For this review, take the finished solid that the model builds, in its own axes (mm). A direction names the side the tool comes from. Give positions to 0.01 mm unless a question says otherwise; leave off trailing zeros. Write each loop counter-clockwise with the first axis right and the second up, starting at its lowest first coordinate (ties: lowest second). Pieces come first, ordered by that corner, then holes.
1) For P1, Ø3, axis at x = 5.5, z = 25, coming from the +Y side; P2, Ø12, axis at x = 18.5, y = 31.5, coming from the +Z side; P3, Ø11, axis at x = -6, z = 17, coming from the +Y side, all flat-tipped, find the tip position at first contact; note any pin that passes through.
2) Machinability: for faces 1 (the face through (34.38, 18.25, 19.14)), 2 (the face through (16, -76.2, 21)), 3 (the face through (38.1, -35, 11)), which of the approach directions +Z, -Z, +X, -X, +Y, -Y give a long, thin tool a straight path to every point of the face, cutting with its end or side? Answer none if there is none.
3) Wall thickness on line 1 along X through (y, z) = (43, 11.5); line 2 along Z through (x, y) = (4, -18); line 3 along Y through (x, z) = (-13, 43): over which ranges is each line inside the solid? List them lowest first.
4) We need section A-A on z = 33. Give the boundary of the cut face in (x, y).
5) We need section D-D on z = 17.5. Give the boundary of the cut face in (x, y), and give its area (3 significant figures).
from build123d import *

# Parameters (mm, degrees)
F0_W        = 88.9
F0_H        = 165.1
F1_DEPTH    = 6.35
F2_DEPTH    = 25.4
F3_DEPTH    = 50.8
F4_R        = 6.34999
F5_C1_SIZE2 = 12.7
F5_C1_SIZE  = 7.3323484187
F5_C2_SIZE2 = 7.3323484187
F5_C2_SIZE  = 12.7
F5_C3_SIZE2 = 7.3323484187
F5_C3_SIZE  = 12.7
F5_C4_SIZE2 = 7.3323484187
F5_C4_SIZE  = 12.7
F5_C5_SIZE2 = 7.3323484187
F5_C5_SIZE  = 12.7
F5_C6_SIZE2 = 7.3323484187
F5_C6_SIZE  = 12.7
F5_C7_SIZE2 = 12.7
F5_C7_SIZE  = 7.3323484187
F6_SIZE2    = 7.3323484187
F6_SIZE     = 12.7


# Not quite as in the source:
# - a fillet or chamfer is up to 0.001 mm smaller than in the source, because OpenCascade refuses the exact size


with BuildPart() as f1:
    # F0 (on Top) → F1 (new body)
    with BuildSketch(Plane.XY):
        Rectangle(F0_W, F0_H)
        Polygon((-38.1, 38.1), (-38.1, 76.2), (0, 76.2), (38.1, 76.2), (38.1, -38.1), (38.1, -76.2), (0, -76.2), (-38.1, -76.2), align=None, mode=Mode.SUBTRACT)
    extrude(amount=F1_DEPTH)

    # F0 (on Top) → F2 (join)
    with BuildSketch(Plane.XY):
        with BuildLine():
            Line((38.1, 76.2), (0, 76.2))
            Line((0, 76.2), (0, 50.8))
            ThreePointArc((0, 50.8), (-3.7197438789, 41.8197438789), (-12.7, 38.1))
            Line((-12.7, 38.1), (-38.1, 38.1))
            Line((-38.1, 38.1), (-38.1, -76.2))
            Line((-38.1, -76.2), (0, -76.2))
            Line((0, -76.2), (0, -50.8))
            ThreePointArc((0, -50.8), (3.7197438789, -41.8197438789), (12.7, -38.1))
            Line((12.7, -38.1), (38.1, -38.1))
            Line((38.1, -38.1), (38.1, 76.2))
        make_face()
    extrude(amount=F2_DEPTH)

    # F0 (on Top) → F3 (join)
    with BuildSketch(Plane.XY):
        with BuildLine():
            Line((38.1, -76.2), (38.1, -38.1))
            Line((38.1, -38.1), (12.7, -38.1))
            ThreePointArc((12.7, -38.1), (3.7197438789, -41.8197438789), (0, -50.8))
            Line((0, -50.8), (0, -76.2))
            Line((0, -76.2), (38.1, -76.2))
        make_face()
        with BuildLine():
            Line((0, 76.2), (-38.1, 76.2))
            Line((-38.1, 76.2), (-38.1, 38.1))
            Line((-38.1, 38.1), (-12.7, 38.1))
            ThreePointArc((-12.7, 38.1), (-3.7197438789, 41.8197438789), (0, 50.8))
            Line((0, 50.8), (0, 76.2))
        make_face()
    extrude(amount=F3_DEPTH)

    # F4 (radius 6.35 in the source; OpenCascade refuses exactly that, so slightly less here)
    f4_edges = [f1.edges().sort_by_distance(p)[0] for p in [
        (0, -82.55, 6.35),
        (44.45, 0, 6.35),
        (0, 82.55, 6.35),
        (-44.45, 0, 6.35),
    ]]
    fillet(f4_edges, radius=F4_R)

    # F5: chamfer of 12.7 x 7.3323484187 on 7 edges, made by hand

    # F5_c1
    f5_c1_edges = [f1.edges().sort_by_distance(p)[0] for p in [
        (-38.1, 57.15, 50.8),
    ]]
    f5_c1_side = f1.faces().sort_by_distance((-38.1, 57.15, 50.6533530316))[0]
    chamfer(f5_c1_edges, length=F5_C1_SIZE, length2=F5_C1_SIZE2, reference=f5_c1_side)

    # F5_c2
    f5_c2_edges = [f1.edges().sort_by_distance(p)[0] for p in [
        (-38.1, -19.05, 25.4),
    ]]
    f5_c2_side = f1.faces().sort_by_distance((-38.1, -19.05, 25.2533530316))[0]
    chamfer(f5_c2_edges, length=F5_C2_SIZE, length2=F5_C2_SIZE2, reference=f5_c2_side)

    # F5_c3
    f5_c3_edges = [f1.edges().sort_by_distance(p)[0] for p in [
        (19.05, 76.2, 25.4),
    ]]
    f5_c3_side = f1.faces().sort_by_distance((19.05, 76.2, 25.2533530316))[0]
    chamfer(f5_c3_edges, length=F5_C3_SIZE, length2=F5_C3_SIZE2, reference=f5_c3_side)

    # F5_c4
    f5_c4_edges = [f1.edges().sort_by_distance(p)[0] for p in [
        (38.1, -57.15, 50.8),
    ]]
    f5_c4_side = f1.faces().sort_by_distance((38.1, -57.15, 50.6533530316))[0]
    chamfer(f5_c4_edges, length=F5_C4_SIZE, length2=F5_C4_SIZE2, reference=f5_c4_side)

    # F5_c5
    f5_c5_edges = [f1.edges().sort_by_distance(p)[0] for p in [
        (38.1, 15.3838257906, 25.4),
    ]]
    f5_c5_side = f1.faces().sort_by_distance((38.1, 15.3838257906, 25.2533530316))[0]
    chamfer(f5_c5_edges, length=F5_C5_SIZE, length2=F5_C5_SIZE2, reference=f5_c5_side)

    # F5_c6
    f5_c6_edges = [f1.edges().sort_by_distance(p)[0] for p in [
        (-15.3838257906, -76.2, 25.4),
    ]]
    f5_c6_side = f1.faces().sort_by_distance((-15.3838257906, -76.2, 25.2533530316))[0]
    chamfer(f5_c6_edges, length=F5_C6_SIZE, length2=F5_C6_SIZE2, reference=f5_c6_side)

    # F5_c7
    f5_c7_edges = [f1.edges().sort_by_distance(p)[0] for p in [
        (15.3838257906, -76.2, 50.8),
    ]]
    f5_c7_side = f1.faces().sort_by_distance((15.3838257906, -76.2, 50.6533530316))[0]
    chamfer(f5_c7_edges, length=F5_C7_SIZE, length2=F5_C7_SIZE2, reference=f5_c7_side)

    # F6
    f6_edges = [f1.edges().sort_by_distance(p)[0] for p in [
        (-12.7, 76.2, 50.8),
    ]]
    f6_side = f1.faces().sort_by_distance((-13.065864, 57.751409, 50.8))[0]
    chamfer(f6_edges, length=F6_SIZE, length2=F6_SIZE2, reference=f6_side)


solid = f1.part
Results list:
1. P1: stops at y = 69.96
1. P2: stops at z = 25.4
1. P3: stops at y = 76.2
2. face 1: +Z, +X, +Y
2. face 2: +Z, +X, -X, -Y
2. face 3: +Z, +X, +Y, -Y
3. line 1: x = -38.1 to 38.1
3. line 2: z = 0 to 25.4
3. line 3: y = 38.1 to 76.2
4. outline: (-38.1, 38.1) - (-12.7, 38.1) arc R12.7 ccw to (0, 50.8) - (0, 76.2) - (-38.1, 76.2) - close; (0, -76.2) - (38.1, -76.2) - (38.1, -38.1) - (12.7, -38.1) arc R12.7 ccw to (0, -50.8) - close
5. outline: (-38.1, 38.1) - (-35.33, 38.1) - (-35.33, -73.43) - (0, -73.43) - (0, -76.2) - (38.1, -76.2) - (38.1, -38.1) - (35.33, -38.1) - (35.33, 73.43) - (0, 73.43) - (0, 76.2) - (-38.1, 76.2) - close
5. area: 10,800 mm2
